Verification items for the finished model (mm, model axes). A direction names the side the tool comes from. Round coordinates to 2 decimals unless told otherwise and drop trailing zeros. Loops run counter-clockwise (first coordinate to the right, second up) from the corner with the lowest first, then second, coordinate; pieces in that order, holes last. Notation, with made-up numbers: (79, 0.25) - (100, 0.25) arc R16 cw to (100, 6.25) - close; hole circle Ø5 at (59.5, 20.25). An arc over 180 degrees is marked (long way). Use CSV: the item, a comma, the result in double quotes.
```python
from build123d import *

# Parameters (mm, degrees)
BOSS_EXTRUDE1_DEPTH            = 40
SKETCH2_W                      = 40
SKETCH2_H                      = 30
BOSS_EXTRUDE2_DEPTH            = 20
BOSS_EXTRUDE3_DEPTH            = 30
CUT_EXTRUDE1_DEPTH             = 30
SKETCH5_W                      = 70
SKETCH5_H                      = 40
BOSS_EXTRUDE4_DEPTH            = 10
SKETCH6_W                      = 20
SKETCH6_H                      = 20
CUT_EXTRUDE2_DEPTH             = 41
F_10_0_10_DIAMETER_HOLE1_D     = 10
F_10_0_10_DIAMETER_HOLE1_DEPTH = 40
FILLET1_R                      = 20


with BuildPart() as part:
    # Sketch1 → Boss-Extrude1 (new body)
    with BuildSketch(Plane(origin=(0, 0, 0), x_dir=(0, -1, 0), z_dir=(-1, 0, 0))):
        Polygon((-10, -2), (-40, -20), (-10, -20), align=None)
    extrude(amount=-BOSS_EXTRUDE1_DEPTH)

    # Sketch2 → Boss-Extrude2 (add)
    with BuildSketch(Plane(origin=(0, 0, -20), x_dir=(-1, 0, 0), z_dir=(0, 0, -1))):
        with Locations((-20, 25)):
            Rectangle(SKETCH2_W, SKETCH2_H)
    extrude(amount=BOSS_EXTRUDE2_DEPTH)

    # Sketch3 → Boss-Extrude3 (add)
    with BuildSketch(Plane(origin=(40, 0, 0), x_dir=(0, 0, -1), z_dir=(1, 0, 0))):
        Polygon((40, 10), (0, 10), (20, 40), (40, 40), align=None)
    extrude(amount=BOSS_EXTRUDE3_DEPTH)

    # Sketch4 → Cut-Extrude1 (cut)
    with BuildSketch(Plane(origin=(70, 0, 0), x_dir=(0, 0, -1), z_dir=(1, 0, 0))):
        Polygon((20, 40), (0, 10), (30, 10), (30, 30), (40, 30), (40, 40), align=None)
    extrude(amount=-CUT_EXTRUDE1_DEPTH, mode=Mode.SUBTRACT)

    # Sketch5 → Boss-Extrude4 (add)
    with BuildSketch(Plane.XZ.offset(-10)):
        with Locations((35, -20)):
            Rectangle(SKETCH5_W, SKETCH5_H)
    extrude(amount=BOSS_EXTRUDE4_DEPTH)

    # Sketch6 → Cut-Extrude2 (cut, through all)
    with BuildSketch(Plane(origin=(0, 0, -40), x_dir=(-1, 0, 0), z_dir=(0, 0, -1))):
        with Locations((-20, 30)):
            Rectangle(SKETCH6_W, SKETCH6_H)
    extrude(amount=-CUT_EXTRUDE2_DEPTH, mode=Mode.SUBTRACT)

    # Ø10.0 (10) Diameter Hole1
    with Locations(Plane(origin=(0, 0, 0), x_dir=(-1, 0, 0), z_dir=(0, -1, 0))):
        with Locations((-55, 15)):
            Hole(F_10_0_10_DIAMETER_HOLE1_D / 2, depth=F_10_0_10_DIAMETER_HOLE1_DEPTH)

    # Fillet1
    fillet1_edges = [part.edges().sort_by_distance(p)[0] for p in [
        (70, 30, -35),
    ]]
    fillet(fillet1_edges, radius=FILLET1_R)


solid = part.part
```
1) Cross-section at B-B, the plane z = -15. Record the cut outline in (x, y), then the cut area to 3 significant figures.
Returned:
outline,"(0, 0) - (50, 0) - (50, 10) - (40, 10) - (40, 31.67) - (30, 31.67) - (30, 20) - (10, 20) - (10, 31.67) - (0, 31.67) - close; (60, 0) - (70, 0) - (70, 10) - (60, 10) - close"
area,"1,230 mm²"
2) Gauge pin test, flat ends, axial feed: pin 1 Ø4 at (y, z) = (12.5, -20.5) entering from -X; pin 2 Ø6 at (x, y) = (56, 16) entering from +Z; pin 3 Ø9 at (x, z) = (46, -15.5) entering from +Y; pin 4 Ø11 at (x, z) = (46, -36) entering from +Y. Record the tip position at first contact, or that the pin passes through.
Returned:
pin 1,"stops at x = 0"
pin 2,"stops at z = -30"
pin 3,"stops at y = 10"
pin 4,"stops at y = 30"
3) Cross-section at D-D, the plane z = -32.5. Record the cut outline in (x, y), then the cut area to 3 significant figures.
Returned:
outline,"(0, 0) - (70, 0) - (70, 10) arc R20 ccw to (50, 30) - (40, 30) - (40, 40) - (30, 40) - (30, 20) - (10, 20) - (10, 40) - (0, 40) - close"
area,"2,010 mm²"
4) Mould release check, pull along X, two halves, no side actions. Record for faces 1 (the face through (10, 30, -28)), 2 (the face through (51, 5, -12)), 3 (the face through (0, 16, -25)), 4 (the face through (52, 20, -30)): +X half, -X half, draft (parallel to the pull), parting line (faces both ways), or undercut.
Returned:
face 1,"undercut"
face 2,"undercut"
face 3,"-X half"
face 4,"draft"
5) Access from +Z, -Z, +X, -X, +Y, -Y to the whole of each face (thin tool, end or side, straight path). Record for faces 5 (the face through (50, 10, -11)), 6 (the face through (70, 5, -20)), 7 (the face through (20, 20, -24)), 8 (the face through (45, 30, -35)), 9 (the face through (35, 0, -20)).
Returned:
face 5,"+Z, +X, +Y"
face 6,"+Z, -Z, +X, +Y, -Y"
face 7,"+Z, -Z, +Y"
face 8,"+Z, -Z, +X, +Y"
face 9,"+Z, -Z, +X, -X, -Y"
6) Cross-section at A-A, the plane y = 22. Record the cut outline in (x, z), then the cut area to 3 significant figures.
Returned:
outline,"(0, -40) - (10, -40) - (10, -9.2) - (0, -9.2) - close; (30, -40) - (66, -40) - (66, -30) - (40, -30) - (40, -9.2) - (30, -9.2) - close"
area,"876 mm²"
7) Thickness scan on probe 1 along X at (y, z) = (27, -13); probe 2 along Z at (x, y) = (55, 2); probe 3 along X at (y, z) = (19.5, -19). Record the ranges inside material, lowest first. Write a range as [from, to].
Returned:
probe 1,"x = [0, 10], [30, 40]"
probe 2,"z = [-40, -20], [-10, 0]"
probe 3,"x = [0, 40]"
8) Cross-section at C-C, the plane y = 3. Record the cut outline in (x, z).
Returned:
outline,"(0, -40) - (70, -40) - (70, 0) - (0, 0) - close; hole circle Ø10 at (55, -15)"
